Input: part model. Units: mm. Frame: model coordinates. A direction names the side the tool comes from. Coordinates: 2 decimals unless noted, no trailing zeros. Loops run counter-clockwise (first coordinate to the right, second up) from the corner with the lowest first, then second, coordinate; pieces in that order, holes last.
(1) Section B-B, the plane z = 0.65. Give the number of separate pieces and of enclosed holes in the cut face, then the cut area to 3 significant figures.
(2) Mould query, pull axis Y, two halves, no side actions, for faces 3 (the face through (201.65, -4.43, 0.02)), 4 (the face through (165.943, 7.695, 0.02)), 5 (the face through (189.491, 4, 0)). Classes: released by +Y, released by -Y, zero draft, split by the parting line, or undercut.
(3) Section A-A, the plane x = 173. Return loops of the section in (y, z).
(4) Line query: L1, parallel to X at y = -4, z = 0.75; L2, parallel to Y at x = 208, z = 0.8; L3, parallel to Y at x = 211, z = 0.4. Output: solid intervals per line, ascending.
(5) Contact query for flat-ended pins moving along their axis: P1, Ø1.2, axis at x = 205.09, y = -3.91, coming from the +Z side; P2, Ø1.5, axis at x = 176, z = 1, coming from the -Y side; P3, Ø0.8, axis at x = 204.5, z = -0.5, coming from the -Y side; P4, Ø0.8, axis at y = 4.5, z = 0.5, coming from the -X side. Output: stop coordinate, or through.
(6) Set-up query: faces 1 (the face through (188, 1.994, 0)), 2 (the face through (205.073, -8.326, 0.02)). Return all of +Z, -Z, +X, -X, +Y, -Y with unobstructed straight access to the full face (end or side cutting, diameter ignored); none if empty.
```python
from build123d import *

# Parameters (mm, degrees)
SKETCH_1_R      = 1
SKETCH_1_R_2    = 3
SKETCH_1_W      = 2.8
SKETCH_1_H      = 5
SKETCH_1_W_2    = 2.85
EXTRUDE_1_DEPTH = 1.4


with BuildPart() as part:
    # Эскиз1 → Бобышка-Вытянуть1 (new, symmetric)
    with BuildSketch(Plane.XY):
        with BuildLine():
            ThreePointArc((175.091334091, 16.644787515), (168.620686799, 13.96455765), (165.940456932, 7.493910359))
            ThreePointArc((165.940456932, 7.493910359), (168.620686797, 1.023263065), (175.091334091, -1.656966802))
            add(Edge.make_bspline(
                [(175.091334091, -1.656966802), (177.330680613, -1.588466601), (181.854695323, -1.455127256), (188.663234462, -1.270383377), (194.423908611, -1.128102082), (197.899847219, -1.04871935), (199.091334091, -1.02226769)],
                knots=[0.704401069, 0.704401069, 0.704401069, 0.704401069, 0.730918775, 0.757971338, 0.785017763, 0.79912389, 0.79912389, 0.79912389, 0.79912389], degree=3))
            Line((199.091334091, -1.02226769), (204.279973699, -7.926463493))
            ThreePointArc((204.279973699, -7.926463493), (205.086497755, -8.325660965), (205.887265796, -7.915039218))
            Line((205.887265796, -7.915039218), (211.091334091, -0.78138581))
            add(Edge.make_bspline(
                [(211.091334091, -0.78138581), (215.029550732, -0.71061193), (221.226120504, -0.611852577), (229.617630172, -0.50292618), (236.087353854, -0.431514192), (241.980776913, -0.376520461), (246.558970011, -0.339535886), (249.120490965, -0.321271242), (250, -0.315)],
                knots=[0.846478182, 0.846478182, 0.846478182, 0.846478182, 0.893099152, 0.919831065, 0.945809917, 0.969680601, 0.989589706, 1, 1, 1, 1], degree=3))
            ThreePointArc((250, -0.315), (250.130477272, 0), (250, 0.315))
            add(Edge.make_bspline(
                [(250, 0.315), (249.15566774, 0.545019818), (246.720175698, 1.208516243), (242.391332083, 2.358339053), (236.849761204, 3.787625364), (230.779918279, 5.298008837), (224.455917947, 6.812866028), (218.030543496, 8.291610632), (211.562405045, 9.719735057), (205.072411509, 11.092374932), (198.567970913, 12.407850726), (192.052369914, 13.665297924), (185.527619973, 14.864093303), (179.872800983, 15.850364437), (176.392239334, 16.431323122), (175.091334091, 16.644787515)],
                knots=[0, 0, 0, 0, 0.0101622, 0.029313053, 0.052011605, 0.076619468, 0.101948061, 0.127526132, 0.153184131, 0.178867888, 0.204557903, 0.230245712, 0.255925967, 0.281594302, 0.296903142, 0.296903142, 0.296903142, 0.296903142], degree=3))
        make_face()
        with Locations((205.091334091, -3.906089643)):
            Circle(SKETCH_1_R, mode=Mode.SUBTRACT)
        with Locations((175.091334091, 7.493910357)):
            Circle(SKETCH_1_R_2, mode=Mode.SUBTRACT)
        with Locations((188.091334091, 4.493910357)):
            Rectangle(SKETCH_1_W, SKETCH_1_H, mode=Mode.SUBTRACT)
        with Locations((205.091334091, 4.493910357)):
            Rectangle(SKETCH_1_W_2, SKETCH_1_H, mode=Mode.SUBTRACT)
    extrude(amount=EXTRUDE_1_DEPTH, both=True)


solid = part.part
```
Report:
1. separate pieces: 1
1. enclosed holes: 4
1. area: 869 mm2
2. face 3: released by -Y
2. face 4: split by the parting line
2. face 5: undercut
3. outline: (-1.41, -1.4) - (5.34, -1.4) - (5.34, 1.4) - (-1.41, 1.4) - close; (9.64, -1.4) - (16.4, -1.4) - (16.4, 1.4) - (9.64, 1.4) - close
4. L1: x = 201.33 to 204.1, 206.09 to 208.74
4. L2: y = -5.02 to 10.47
4. L3: y = -0.91 to 9.83
5. P1: passes through
5. P2: stops at y = -1.65
5. P3: stops at y = -8.31
5. P4: stops at x = 166.32
6. face 1: +Z, -Z
6. face 2: +Z, -Z, -Y
